Read the model definition and answer for the solid it produces. Units are mm, in the model's axes. A direction names the side the tool comes from. Give positions to 0.01 mm unless a question says otherwise; leave off trailing zeros. Order: outer loops, then holes, each group sorted by start corner. A loop starts at its lowest first (then second) coordinate and runs counter-clockwise, first axis right, second up. Notation, with made-up numbers: (-9.5, 1.25) - (30.5, 1.25) arc R24 cw to (30.5, 33.25) - close; hole circle Ø9 at (-7, -37.75). An arc over 180 degrees is marked (long way). One line per item, written item: value. Start each with the question number.
```python
from build123d import *

# Parameters (mm, degrees)
SKETCH1_W                    = 110.7186
SKETCH1_H                    = 19.939
BASE_FLANGE1_DEPTH           = 1.016
EDGE_FLANGE1_STRIP_W         = 5.5372
EDGE_FLANGE1_STRIP_H         = 1.016
EDGE_FLANGE1_STRIP_CUT_DEPTH = 110.7186
EDGE_FLANGE1_DEPTH           = 110.7186
CUT_EXTRUDE1_REACH           = 116.94
SKETCH9_W                    = 90.7796
SKETCH9_H                    = 23.6474
EDGE_FLANGE2_STRIP_W         = 5.5372
EDGE_FLANGE2_STRIP_H         = 1.016
EDGE_FLANGE2_STRIP_CUT_DEPTH = 19.939
EDGE_FLANGE2_DEPTH           = 19.939
EDGE_FLANGE3_STRIP_W         = 5.5372
EDGE_FLANGE3_STRIP_H         = 1.016
EDGE_FLANGE3_STRIP_CUT_DEPTH = 19.939
EDGE_FLANGE3_DEPTH           = 19.939
CUT_EXTRUDE2_DEPTH           = 2.54
CUT_EXTRUDE2_DEPTH_BACK      = 2.54
SKETCH17_W                   = 38.49878
SKETCH17_H                   = 1.7526
SKETCH16_W                   = 38.49878
SKETCH16_H                   = 12.7
TAB2_DEPTH                   = 1.016
CUT_EXTRUDE3_REACH           = 128.228
SKETCH20_R                   = 4.2545
CUT_EXTRUDE4_REACH           = 128.58
SKETCH21_R                   = 2.36295848


# Sheet-metal steps are written as plain solids
with BuildPart() as part:
    # Sketch1 → Base-Flange1 (new body)
    with BuildSketch(Plane(origin=(0, 0, 0), x_dir=(1, 0, 0), z_dir=(0, 1, 0))):
        with Locations((-55.3593, 9.9695)):
            Rectangle(SKETCH1_W, SKETCH1_H)
    extrude(amount=-BASE_FLANGE1_DEPTH)

    # Edge-Flange1 strip (across the edge) → Edge-Flange1 strip cut (cut)
    with BuildSketch(Plane(origin=(0, 0, -19.939), x_dir=(0, 0, 1), z_dir=(-1, 0, 0))):
        with Locations((-1.016, -0.508)):
            Rectangle(EDGE_FLANGE1_STRIP_W, EDGE_FLANGE1_STRIP_H)
    extrude(amount=EDGE_FLANGE1_STRIP_CUT_DEPTH, mode=Mode.SUBTRACT)

    # Edge-Flange1 section (across the edge) → Edge-Flange1 (add)
    with BuildSketch(Plane(origin=(0, 0, -19.939), x_dir=(0, 0, 1), z_dir=(-1, 0, 0))):
        with BuildLine():
            Line((0, 0.7366), (0, 24.384))
            Line((0, 24.384), (1.016, 24.384))
            Line((1.016, 24.384), (1.016, 0.7366))
            ThreePointArc((1.016, 0.7366), (1.231745145, 0.215745145), (1.7526, 0))
            Line((1.7526, 0), (1.7526, -1.016))
            ThreePointArc((1.7526, -1.016), (0.513324655, -0.502675345), (0, 0.7366))
        make_face()
    extrude(amount=EDGE_FLANGE1_DEPTH)

    # Sketch9 → Cut-Extrude1 (cut, up to next)
    with BuildSketch(Plane.XY.offset(-18.923), mode=Mode.PRIVATE) as cut_extrude1_sk1:
        with Locations((-45.3898, 12.5603)):
            Rectangle(SKETCH9_W, SKETCH9_H)
    cut_extrude1_tool1 = extrude(cut_extrude1_sk1.sketch, amount=-CUT_EXTRUDE1_REACH, mode=Mode.PRIVATE) & part.part
    add(cut_extrude1_tool1.solids().sort_by_distance((-45.3898, 12.5603, -18.923))[0], mode=Mode.SUBTRACT)

    # Edge-Flange2 strip (across the edge) → Edge-Flange2 strip cut (cut)
    with BuildSketch(Plane(origin=(-110.7186, 24.384, -19.939), x_dir=(0, -1, 0), z_dir=(1, 0, 0))):
        with Locations((-1.016, -0.508)):
            Rectangle(EDGE_FLANGE2_STRIP_W, EDGE_FLANGE2_STRIP_H)
    extrude(amount=EDGE_FLANGE2_STRIP_CUT_DEPTH, mode=Mode.SUBTRACT)

    # Edge-Flange2 section (across the edge) → Edge-Flange2 (add)
    with BuildSketch(Plane(origin=(-110.7186, 24.384, -19.939), x_dir=(0, -1, 0), z_dir=(1, 0, 0))):
        with BuildLine():
            Line((0, 0.7366), (0, 24.384))
            Line((0, 24.384), (1.016, 24.384))
            Line((1.016, 24.384), (1.016, 0.7366))
            ThreePointArc((1.016, 0.7366), (1.231745145, 0.215745145), (1.7526, 0))
            Line((1.7526, 0), (1.7526, -1.016))
            ThreePointArc((1.7526, -1.016), (0.513324655, -0.502675345), (0, 0.7366))
        make_face()
    extrude(amount=EDGE_FLANGE2_DEPTH)

    # Edge-Flange3 strip (across the edge) → Edge-Flange3 strip cut (cut)
    with BuildSketch(Plane(origin=(-90.7796, 24.384, -44.323), x_dir=(0, 0, 1), z_dir=(-1, 0, 0))):
        with Locations((-1.016, -0.508)):
            Rectangle(EDGE_FLANGE3_STRIP_W, EDGE_FLANGE3_STRIP_H)
    extrude(amount=EDGE_FLANGE3_STRIP_CUT_DEPTH, mode=Mode.SUBTRACT)

    # Edge-Flange3 section (across the edge) → Edge-Flange3 (add)
    with BuildSketch(Plane(origin=(-90.7796, 24.384, -44.323), x_dir=(0, 0, 1), z_dir=(-1, 0, 0))):
        with BuildLine():
            Line((0, 0.7366), (0, 18.034))
            Line((0, 18.034), (1.016, 18.034))
            Line((1.016, 18.034), (1.016, 0.7366))
            ThreePointArc((1.016, 0.7366), (1.231745145, 0.215745145), (1.7526, 0))
            Line((1.7526, 0), (1.7526, -1.016))
            ThreePointArc((1.7526, -1.016), (0.513324655, -0.502675345), (0, 0.7366))
        make_face()
    extrude(amount=EDGE_FLANGE3_DEPTH)

    # Sketch17 → Cut-Extrude2 (cut, two sides: drawn at the far end of the back side and taken through both)
    with BuildSketch(Plane(origin=(0, 0, 0), x_dir=(1, 0, 0), z_dir=(0, 1, 0)).offset(-CUT_EXTRUDE2_DEPTH_BACK)):
        with Locations((-19.24939, 19.0627)):
            Rectangle(SKETCH17_W, SKETCH17_H)
    extrude(amount=CUT_EXTRUDE2_DEPTH + CUT_EXTRUDE2_DEPTH_BACK, mode=Mode.SUBTRACT)

    # Sketch16 → Tab2 (add)
    with BuildSketch(Plane(origin=(0, 0, 0), x_dir=(1, 0, 0), z_dir=(0, 1, 0))):
        with Locations((-19.24939, 24.5364)):
            Rectangle(SKETCH16_W, SKETCH16_H)
    extrude(amount=-TAB2_DEPTH)

    # Sketch20 → Cut-Extrude3 (cut, up to next)
    with BuildSketch(Plane.XY.offset(-43.307), mode=Mode.PRIVATE) as cut_extrude3_sk1:
        with Locations((-101.6161, 31.368930224)):
            Circle(SKETCH20_R)
    cut_extrude3_tool1 = extrude(cut_extrude3_sk1.sketch, amount=-CUT_EXTRUDE3_REACH, mode=Mode.PRIVATE) & part.part
    add(cut_extrude3_tool1.solids().sort_by_distance((-101.6161, 31.36893, -43.307))[0], mode=Mode.SUBTRACT)

    # Sketch21 → Cut-Extrude4 (cut, up to next)
    with BuildSketch(Plane(origin=(0, 0, 0), x_dir=(1, 0, 0), z_dir=(0, 1, 0)), mode=Mode.PRIVATE) as cut_extrude4_sk1:
        with Locations(Location((-27.6261, 25.7429, 0), (0, 0, 270))):
            Circle(SKETCH21_R)
    cut_extrude4_tool1 = extrude(cut_extrude4_sk1.sketch, amount=-CUT_EXTRUDE4_REACH, mode=Mode.PRIVATE) & part.part
    # Sketch21 → Cut-Extrude4 (cut, up to next)
    with BuildSketch(Plane(origin=(0, 0, 0), x_dir=(1, 0, 0), z_dir=(0, 1, 0)), mode=Mode.PRIVATE) as cut_extrude4_sk2:
        with Locations(Location((-5.6261, 25.7429, 0), (0, 0, 270))):
            Circle(SKETCH21_R)
    cut_extrude4_tool2 = extrude(cut_extrude4_sk2.sketch, amount=-CUT_EXTRUDE4_REACH, mode=Mode.PRIVATE) & part.part
    add(cut_extrude4_tool1.solids().sort_by_distance((-27.6261, 0, -25.7429))[0], mode=Mode.SUBTRACT)
    add(cut_extrude4_tool2.solids().sort_by_distance((-5.6261, 0, -25.7429))[0], mode=Mode.SUBTRACT)


solid = part.part
```
1) Section B-B on x = -82.5 is taken. Write down the section's boundary in (y, z), plus the area to 3 significant figures.
2) For faces 5 (the flat face through (-110.719, 24, -29)), 6 (the flat face through (-101, 36, -43.307)), 7 (the flat face through (-101, 12, -19.939)), 8 (the flat face through (-44, -1.016, -12)), 9 (the flat face through (-90.78, 21.7, -19.3)), determine the directions among +Z, -Z, +X, -X, +Y, -Y from which every point of the face is accessible in a straight line to the end or side of a thin tool.
3) Section C-C on z = -6.5 is taken. Write down the section's boundary in (x, y), plus the area to 3 significant figures.
4) Section A-A on z = -26 is taken. Write down the section's boundary in (x, y), plus the area to 3 significant figures.
5) Section D-D on y = 20.5 is taken. Write down the section's boundary in (x, z), plus the area to 3 significant figures.
6) Find the intervals of material crossed by probe 1 along Y at (x, z) = (-79, -14); probe 2 along Y at (x, z) = (-100.5, -26); probe 3 along Z at (x, y) = (-94, 21), in increasing order. Write a range as from..to.
7) Each of these flat-tipped pins is pushed along its axis until it touches: pin 1 (0.8 mm diameter, centred on y = -0.5, z = -26, fed in from -X); pin 2 (14 mm diameter, centred on x = -100.5, y = 31, fed in from +Z); pin 3 (0.5 mm diameter, centred on x = -57.5, z = -19.5, fed in from +Y). Where does it stop, or does it pass through?
8) The mould has two halves that part along Z. Classify faces 1 (the flat face through (-44, 0, -12)), 2 (the cylindrical face through (-29.72, -0.5, -24.65)), 3 (the flat face through (-101, 12, -18.923)), 4 (the cylindrical face through (-4.92, -0.5, -23.49)): +Z half, -Z half, draft (parallel to the pull), parting line (faces both ways), or undercut.
Solved:
1. outline: (-1.02, -18.19) arc R1.75 ccw to (0.74, -19.94) - (0.74, -18.92) arc R0.74 cw to (0, -18.19) - (0, 0) - (-1.02, 0) - close
1. area: 20.5 mm2
2. face 5: +Z, -Z, -X, +Y, -Y
2. face 6: +Z, +X, -X, +Y
2. face 7: -Z, +X, -X, -Y
2. face 8: +Z, -Z, +X, -X, -Y
2. face 9: +Z, -Z, +X, +Y
3. outline: (-110.72, -1.02) - (0, -1.02) - (0, 0) - (-110.72, 0) - close
3. area: 112 mm2
4. outline: (-110.72, 23.37) - (-90.78, 23.37) - (-90.78, 24.38) - (-110.72, 24.38) - close; (-38.5, -1.02) - (-29.98, -1.02) - (-29.98, 0) - (-38.5, 0) - close; (-25.28, -1.02) - (-7.98, -1.02) - (-7.98, 0) - (-25.28, 0) - close; (-3.28, -1.02) - (0, -1.02) - (0, 0) - (-3.28, 0) - close
4. area: 49.8 mm2
5. outline: (-110.72, -19.94) - (-90.78, -19.94) - (-90.78, -18.92) - (-110.72, -18.92) - close
5. area: 20.3 mm2
6. probe 1: y = -1.02..0
6. probe 2: y = 23.37..24.38
6. probe 3: z = -19.94..-18.92
7. pin 1: stops at x = -38.5
7. pin 2: stops at z = -19.58
7. pin 3: stops at y = 0.74
8. face 1: draft
8. face 2: undercut
8. face 3: +Z half
8. face 4: undercut
